Could you check a few things on this drawing? It's one solid part, dimensions in mm from its lowest x, y, z. Coordinates: 2 decimals unless noted, no trailing zeros. Write each loop counter-clockwise with the first axis right and the second up, starting at its lowest first coordinate (ties: lowest second). Pieces come first, ordered by that corner, then holes.
Item 1: I want a section at A-A (y = 4.5). Please give me the cut outline in (x, z).
Item 2: Please list where these lines run through material, in increasing order: line 1 (X direction, y = 10.5, z = 67.29); line 2 (Y direction, x = 22, z = 7.5); line 3 (X direction, y = 6, z = 102).
Item 3: I'm going to push flat-ended pins straight in: P1, Ø0.9, axis at x = 2, y = 4.5, coming from the +Z side; P2, Ø4, axis at x = 67.06, z = 67.29, coming from the -Y side; P3, Ø2.5, axis at x = 1.5, y = 3, coming from the -Z side. Where does each tip first touch, or does it pass through?
Item 4: I want a section at B-B (z = 67.29). Please give me the cut outline in (x, y).
Item 5: I want a section at C-C (x = 59). Please give me the cut outline in (y, z), and give its area (3 significant figures).
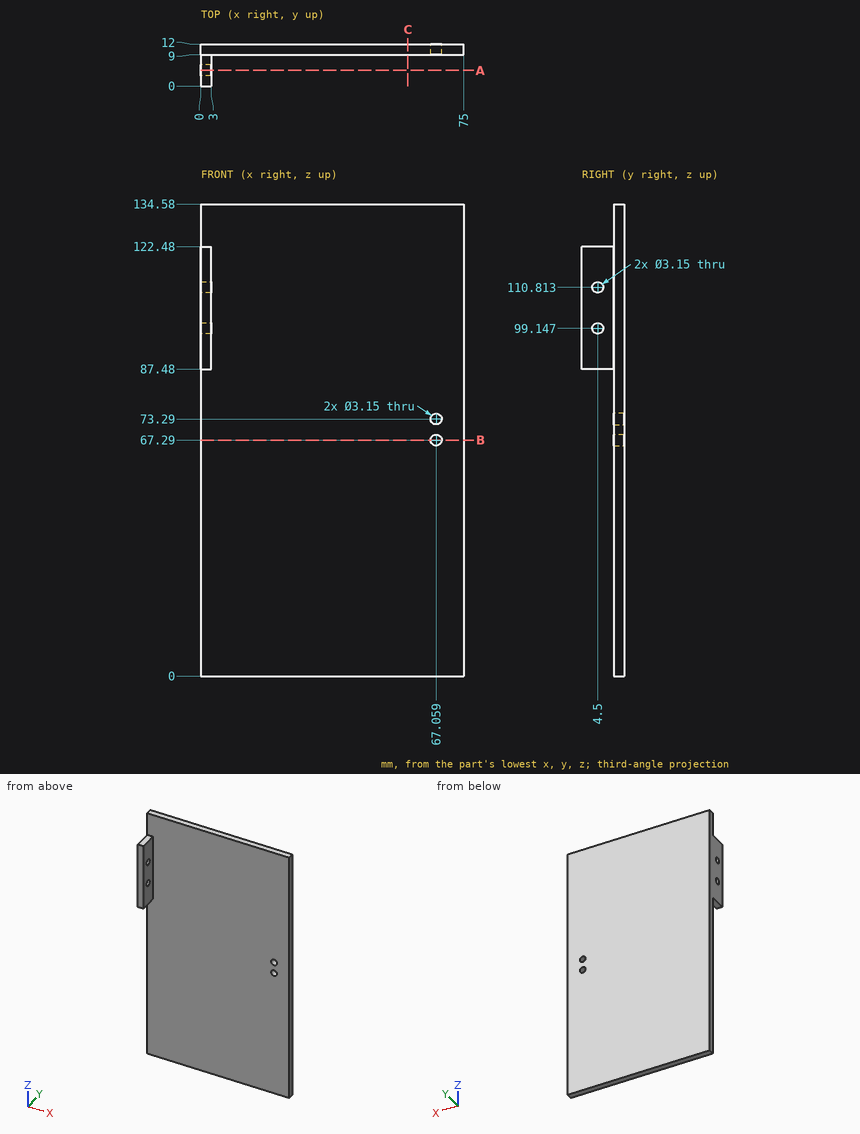
Answer:
1. outline: (0, 87.48) - (3, 87.48) - (3, 97.57) - (0, 97.57) - close; (0, 100.72) - (3, 100.72) - (3, 109.24) - (0, 109.24) - close; (0, 112.39) - (3, 112.39) - (3, 122.48) - (0, 122.48) - close
2. line 1: x = 0 to 65.48, 68.63 to 75
2. line 2: y = 9 to 12
2. line 3: x = 0 to 3
3. P1: stops at z = 122.48
3. P2: stops at y = 9
3. P3: stops at z = 87.48
4. outline: (0, 9) - (65.48, 9) - (65.48, 12) - (0, 12) - close; (68.63, 9) - (75, 9) - (75, 12) - (68.63, 12) - close
5. outline: (9, 0) - (12, 0) - (12, 134.58) - (9, 134.58) - close
5. area: 404 mm2
